Work out the finished part from the listing and answer in its coordinate system (mm). A direction names the side the tool comes from. Coordinates: 2 decimals unless noted, no trailing zeros. Order: outer loops, then holes, each group sorted by start corner. A loop starts at its lowest first (then second) coordinate and runs counter-clockwise, first axis right, second up. Notation, with made-up numbers: (42, -38.75) -> (58, -38.75) arc R21 cw to (58, -1.75) -> close; hole circle Ø3 at (67.25, -13). An arc over 180 degrees is marked (long way). Answer as CSV lines item,"result". Start each with the question number.
Item 1: Which of the six approach directions +Z, -Z, +X, -X, +Y, -Y give full straight-line access (tool end or side, diameter ignored) to faces 1 (the face through (-89.88, 10.61, 38.24)), 2 (the face through (-54, 3, 67.16)), 3 (the face through (-92.257, 5, 49))?
Item 2: For a pull along X with two mould halves and no side action, classify faces 4 (the face through (-93, 1.896, 60)), 5 (the face through (-55.257, 3, 62)), 6 (the face through (-92.257, 4, 60)) as pulls with the +X half, pulls with the -X half, needs draft (parallel to the pull), parting line crosses it, or undercut.
Item 3: Straight lines are drawn through the part: L1, parallel to Z at x = -71.5, y = 8; L2, parallel to X at y = 1.25, z = 71.5; L3, parallel to Z at x = -89, y = 6.25. For each, find the intervals that lie inside material, in ascending order.
Item 4: Section A-A (y = 15) is taken. Write down the section's boundary in (x, z).
Item 5: Section C-C (x = -68) is taken. Write down the section's boundary in (y, z).
Item 6: Each of these flat-tipped pins is pushed along its axis until it touches: pin 1 Ø2 at (y, z) = (11.5, 49) entering from -X; pin 2 Ø6 at (x, y) = (-65.5, 11.5) entering from +Z; pin 3 Ø4 at (x, z) = (-88, 46) entering from +Y. Where does it stop, or does it pass through?
Item 7: Section B-B (y = 11) is taken. Count the separate pieces of the cut face and the enclosed holes in it, then the cut area to 3 significant figures.
Autodesk Inventor part; units mm, degrees
ref_plane "YZ Plane" through (0, 0, 0) normal (1, 0, 0) x (0, 1, 0)
ref_plane "XZ Plane" through (0, 0, 0) normal (0, 1, 0) x (-1, 0, 0)
ref_plane "XY Plane" through (0, 0, 0) normal (0, 0, 1) x (1, 0, 0)
sketch "Sketch1" plane through (0, 0, 0) normal (0, 1, 0) x (-1, 0, 0)
  line L0 (94.2568, 73.4599) -> (94.2568, 30.8599)
  line L1 (94.2568, 30.8599) -> (50.7568, 30.8599)
  line L2 (50.7568, 30.8599) -> (50.7568, 73.4599)
  line L3 (50.7568, 73.4599) -> (94.2568, 73.4599)
  point P0 (0, 0)
  dimension "d0" = 42.6
  dimension "d1" = 43.5
extrude "Extrusion1" add sketch "Sketch1" along normal blind 1.6
sketch "Sketch2" plane through (0, 1.6, 0) normal (0, 1, 0) x (1, 0, 0)
  circle A0 centre (-53.6568, -70.5599) radius 1.5
  circle A1 centre (-53.6568, -33.9599) radius 1.5
  line L0 (-94.2568, -73.4599) -> (-50.7568, -73.4599)
  line L1 (-50.7568, -73.4599) -> (-50.7568, -30.8599)
  circle A2 centre (-91.6568, -33.9599) radius 1.5
  circle A3 centre (-91.6568, -70.5599) radius 1.5
  line L2 (-94.2568, -30.8599) -> (-94.2568, -73.4599)
  point P0 (0, 0)
  dimension "d4" = 3
  dimension "d5" = 3
  dimension "d6" = 36.6
  dimension "d7" = 2.9
  dimension "d8" = 2.9
  dimension "d9" = 2.9
  dimension "d10" = 3
  dimension "d11" = 38
  dimension "d12" = 3
  dimension "d13" = 38
  dimension "d14" = 2.6
extrude "Extrusion2" cut sketch "Sketch2" against normal blind 1.6
sketch "Sketch3" plane through (0, 1.6, 0) normal (0, 1, 0) x (1, 0, 0)
  line L0 (-65.7568, -67.8599) -> (-65.7568, -52.8599)
  line L1 (-65.7568, -51.8599) -> (-65.7568, -36.8599)
  line L2 (-50.7568, -73.4599) -> (-50.7568, -30.8599)
  line L3 (-65.7568, -67.8599) -> (-84.5568, -67.8599)
  line L4 (-84.5568, -67.8599) -> (-84.5568, -52.8599)
  line L5 (-84.5568, -52.8599) -> (-65.7568, -52.8599)
  line L6 (-65.7568, -51.8599) -> (-84.5568, -51.8599)
  line L7 (-84.5568, -51.8599) -> (-84.5568, -36.8599)
  line L8 (-84.5568, -36.8599) -> (-65.7568, -36.8599)
  line L9 (-94.2568, -73.4599) -> (-50.7568, -73.4599)
  point P0 (0, 0)
  dimension "d17" = 15
  dimension "d18" = 15
  dimension "d19" = 15
  dimension "d20" = 15
  dimension "d21" = 18.8
  dimension "d22" = 5.6
  dimension "d23" = 1
sketch "Sketch4" plane through (0, 1.6, 0) normal (0, 1, 0) x (1, 0, 0)
  line L0 (-55.2568, -67.1599) -> (-55.2568, -57.1599)
  line L1 (-55.2568, -57.1599) -> (-52.7568, -57.1599)
  line L2 (-52.7568, -57.1599) -> (-52.7568, -67.1599)
  line L3 (-52.7568, -67.1599) -> (-55.2568, -67.1599)
  line L4 (-50.7568, -73.4599) -> (-50.7568, -30.8599)
  line L5 (-94.2568, -73.4599) -> (-50.7568, -73.4599)
  point P0 (0, 0)
  dimension "d26" = 10
  dimension "d27" = 2
  dimension "d28" = 2.5
  dimension "d29" = 6.3
extrude "Extrusion4" add sketch "Sketch4" along normal blind 3
sketch "Sketch5" plane through (0, 4.6, 0) normal (0, 1, 0) x (1, 0, 0)
  circle A0 centre (-54.0568, -65.3099) radius 0.3
  circle A1 centre (-54.0568, -63.2099) radius 0.3
  circle A2 centre (-54.0568, -61.1099) radius 0.3
  circle A3 centre (-54.0568, -59.0099) radius 0.3
  line L0 (-55.2568, -67.1599) -> (-52.7568, -67.1599)
  line L1 (-52.7568, -67.1599) -> (-52.7568, -57.1599)
  point P0 (0, 0)
  dimension "d32" = 0.6
  dimension "d33" = 0.6
  dimension "d34" = 0.6
  dimension "d35" = 0.6
  dimension "d36" = 1.85
  dimension "d37" = 1.3
  dimension "d38" = 2.1
  dimension "d39" = 2.1
  dimension "d40" = 2.1
  dimension "d41" = 1.3
extrude "Extrusion5" add sketch "Sketch5" along normal blind 5.8
sketch "Sketch6" plane through (0, 1.6, 0) normal (0, 1, 0) x (1, 0, 0)
  circle A0 centre (-54.0568, -38.8599) radius 2
  circle A1 centre (-54.0568, -47.2599) radius 2
  circle A2 centre (-54.0568, -52.7599) radius 2
  circle A3 centre (-53.6568, -33.9599) radius 1.5
  line L0 (-50.7568, -30.8599) -> (-94.2568, -30.8599)
  line L1 (-50.7568, -30.8599) -> (-50.7568, -73.4599)
  point P0 (0, 0)
  dimension "d44" = 4
  dimension "d45" = 4
  dimension "d46" = 4
  dimension "d48" = 8
  dimension "d49" = 8.4
  dimension "d50" = 5.5
  dimension "d51" = 3.3
extrude "Extrusion6" add sketch "Sketch6" along normal blind 1.2 contours A0 | A1 | A2
sketch "Sketch7" plane through (-54.0568, 2.8, 52.7599) normal (0, 1, 0) x (1, 0, 0)
  circle A0 centre (0, 0) radius 2
  circle A1 centre (0, 0) radius 1.5
  point P0 (54.0568, 52.7599)
  dimension "d54" = 3
sketch "Sketch8" plane through (-54.0568, 2.8, 47.2599) normal (0, 1, 0) x (1, 0, 0)
  circle A0 centre (0, 0) radius 2
  circle A1 centre (0, 0) radius 1.5
  point P0 (54.0568, 47.2599)
  dimension "d55" = 3
sketch "Sketch9" plane through (-54.0568, 2.8, 38.8599) normal (0, 1, 0) x (1, 0, 0)
  circle A0 centre (0, 0) radius 2
  circle A1 centre (0, 0) radius 1.5
  point P0 (54.0568, 38.8599)
  dimension "d56" = 3
extrude "Extrusion7" add sketch "Sketch7" along normal blind 4.3 contours A1
extrude "Extrusion8" add sketch "Sketch8" along normal blind 4.3 contours A1
extrude "Extrusion9" add sketch "Sketch9" along normal blind 4.3 contours A1
fillet "Fillet1" radius 1.5 3 edges at (-55.5568, 7.1, 52.7599) (-55.5568, 7.1, 47.2599) (-55.5568, 7.1, 38.8599)
sketch "Sketch10" plane through (0, 1.6, 0) normal (0, 1, 0) x (1, 0, 0)
  line L0 (-85.2568, -36.9599) -> (-85.2568, -51.9599)
  line L1 (-85.2568, -51.9599) -> (-93.2568, -51.9599)
  line L2 (-93.2568, -51.9599) -> (-93.2568, -36.9599)
  line L3 (-93.2568, -36.9599) -> (-85.2568, -36.9599)
  line L4 (-93.2568, -52.9599) -> (-85.2568, -52.9599)
  line L5 (-85.2568, -52.9599) -> (-85.2568, -67.9599)
  line L6 (-85.2568, -67.9599) -> (-93.2568, -67.9599)
  line L7 (-93.2568, -67.9599) -> (-93.2568, -52.9599)
  line L8 (-84.5568, -36.8599) -> (-84.5568, -51.8599)
  line L9 (-50.7568, -30.8599) -> (-94.2568, -30.8599)
  point P0 (0, 0)
  dimension "d64" = 8
  dimension "d65" = 0.7
  dimension "d66" = 6.1
  dimension "d67" = 15
  dimension "d68" = 15
  dimension "d69" = 1
extrude "Extrusion10" add sketch "Sketch10" along normal blind 6
sketch "Sketch11" plane through (-93.2568, 1.6, 36.9599) normal (-1, 0, 0) x (0, 0, 1)
  line L0 (0.4, 0.8) -> (0.4, 5.8)
  line L1 (0.4, 5.8) -> (4.7, 5.8)
  line L2 (4.7, 5.8) -> (4.7, 0.8)
  line L3 (4.7, 0.8) -> (0.4, 0.8)
  line L4 (15, 0) -> (0, 0)
  line L5 (5.3, 5.8) -> (9.6, 5.8)
  line L6 (9.6, 5.8) -> (9.6, 0.8)
  line L7 (9.6, 0.8) -> (5.3, 0.8)
  line L8 (5.3, 0.8) -> (5.3, 5.8)
  line L9 (10.2, 5.8) -> (14.5, 5.8)
  line L10 (14.5, 5.8) -> (14.5, 0.8)
  line L11 (14.5, 0.8) -> (10.2, 0.8)
  line L12 (10.2, 0.8) -> (10.2, 5.8)
  line L13 (0, 0) -> (0, 6)
  point P0 (-36.9599, -1.6)
  dimension "d72" = 4.3
  dimension "d73" = 5
  dimension "d74" = 0.8
  dimension "d75" = 4.3
  dimension "d76" = 4.3
  dimension "d77" = 5
  dimension "d78" = 0.6
  dimension "d79" = 0.6
  dimension "d80" = 0.4
extrude "Extrusion11" cut sketch "Sketch11" against normal blind 1
sketch "Sketch12" plane through (0, 7.6, 0) normal (0, 1, 0) x (1, 0, 0)
  line L0 (-86.0568, -36.9599) -> (-91.0568, -36.9599)
  line L1 (-92.2568, -47.1599) -> (-92.2568, -51.4599)
  line L2 (-92.2568, -51.9599) -> (-86.0568, -51.9599)
  line L3 (-86.0568, -51.9599) -> (-86.0568, -36.9599)
  line L4 (-85.2568, -36.9599) -> (-93.2568, -36.9599)
  line L5 (-93.2568, -51.9599) -> (-85.2568, -51.9599)
  line L6 (-84.5568, -36.8599) -> (-84.5568, -51.8599)
  line L7 (-91.0568, -36.9599) -> (-91.0568, -51.9599)
  line L8 (-86.0568, -36.9599) -> (-91.0568, -36.9599)
  line L9 (-86.0568, -51.9599) -> (-91.0568, -51.9599)
  point P0 (0, 0)
  dimension "d83" = 0
  dimension "d84" = 0
  dimension "d85" = 1.5
  dimension "d86" = 5
extrude "Extrusion12" add sketch "Sketch12" along normal blind 4
ref_plane "Work Plane2" through (-91.0568, 11.6, 36.9599) normal (0.8762, -0.4819, 0) x (0, 0, 1)
sketch "Sketch13" plane through (-91.0568, 11.6, 36.9599) normal (0.8762, -0.4819, 0) x (0, 0, 1)
  line L0 (0, 0) -> (0, 4.5651)
  line L1 (0, 5.967) -> (0, 0.7097)
  line L2 (0, 4.5651) -> (15, 4.5651)
  line L3 (0, 4.5651) -> (15, 4.5651)
  line L4 (15, 4.5651) -> (15, 0)
  line L5 (15, 0) -> (0, 0)
  line L6 (0, 0) -> (15, 0)
  point P0 (-36.9599, -33.7179)
extrude "Extrusion13" add sketch "Sketch13" along normal blind 2
ref_plane "Work Plane3" through (-86.0568, 11.6, 51.9599) normal (-0.9806, -0.1961, 0) x (0, 0, -1)
sketch "Sketch14" plane through (-86.0568, 11.6, 51.9599) normal (-0.9806, -0.1961, 0) x (0, 0, -1)
  line L0 (15, 0) -> (15, 4.0792)
  line L1 (15, 4.0792) -> (0, 4.0792)
  line L2 (0, 4.0792) -> (0, 0)
  line L3 (0, 0) -> (15, 0)
  line L4 (0, 0) -> (15, 0)
  point P0 (51.9599, 28.2519)
extrude "Extrusion14" add sketch "Sketch14" along normal blind 2
sketch "Sketch15" plane through (0, 11.6, 0) normal (0, 1, 0) x (1, 0, 0)
  circle A0 centre (-88.5568, -39.4599) radius 1.8
  circle A1 centre (-88.5568, -44.4599) radius 1.8
  circle A2 centre (-88.5568, -49.4599) radius 1.8
  line L0 (-86.0568, -36.9599) -> (-91.0568, -36.9599)
  line L1 (-91.0568, -51.9599) -> (-86.0568, -51.9599)
  point P0 (0, 0)
  dimension "d93" = 3.6
  dimension "d94" = 3.6
  dimension "d95" = 3.6
  dimension "d96" = 2.5
  dimension "d97" = 5
  dimension "d98" = 5
extrude "Extrusion15" cut sketch "Sketch15" against normal blind 2
sketch "Sketch16" plane through (0, 7.6, 0) normal (0, 1, 0) x (1, 0, 0)
  line L0 (-85.2568, -52.9599) -> (-86.0568, -52.9599)
  line L1 (-85.2568, -52.9599) -> (-93.2568, -52.9599)
  line L2 (-86.0568, -51.9599) -> (-86.0568, -36.9599)
  line L3 (-86.0568, -52.9599) -> (-91.0568, -52.9599)
  line L4 (-91.0568, -52.9599) -> (-91.0568, -67.9599)
  line L5 (-93.2568, -67.9599) -> (-85.2568, -67.9599)
  line L6 (-86.0568, -52.9599) -> (-86.0568, -67.9599)
  line L7 (-91.0568, -67.9599) -> (-86.0568, -67.9599)
  point P0 (0, 0)
  dimension "d102" = 5
extrude "Extrusion16" add sketch "Sketch16" along normal blind 4
sketch "Sketch17" plane through (-91.0568, 11.6, 36.9599) normal (0.8762, -0.4819, 0) x (0, 0, 1)
  line L0 (16, 0) -> (16, 4.5662)
  line L1 (16, 4.5662) -> (31, 4.5662)
  line L2 (31, 5.967) -> (31, 0.7097)
  line L3 (31, 4.5662) -> (31, 0)
  line L4 (31, 1.0953) -> (31, -2.4096)
  line L5 (31, 0) -> (16, 0)
  line L6 (16, 0) -> (31, 0)
  point P0 (-36.9599, -33.7179)
extrude "Extrusion17" add sketch "Sketch17" along normal blind 4
sketch "Sketch18" plane through (-86.0568, 11.6, 51.9599) normal (-0.9806, -0.1961, 0) x (0, 0, -1)
  line L0 (-1, 4.0792) -> (-1, 0)
  line L1 (-1, 0) -> (-16, 0)
  line L2 (-16, 0) -> (-1, 0)
  line L3 (-16, 0) -> (-16, 4.0792)
  line L4 (-16, 3.9223) -> (-16, 0)
  line L5 (-16, 4.0792) -> (-1, 4.0792)
  line L6 (-16, 4.0792) -> (-1, 4.0792)
  point P0 (51.9599, 28.2519)
extrude "Extrusion18" add sketch "Sketch18" along normal blind 4
sketch "Sketch19" plane through (0, 11.6, 0) normal (0, 1, 0) x (1, 0, 0)
  circle A0 centre (-88.5568, -55.4599) radius 1.8
  circle A1 centre (-88.5568, -60.4599) radius 1.8
  circle A2 centre (-88.5568, -65.4599) radius 1.8
  line L0 (-86.0568, -52.9599) -> (-91.0568, -52.9599)
  line L1 (-91.0568, -67.9599) -> (-86.0568, -67.9599)
  line L2 (-91.0568, -52.9599) -> (-91.0568, -67.9599)
  point P0 (0, 0)
  dimension "d109" = 3.6
  dimension "d110" = 3.6
  dimension "d111" = 3.6
  dimension "d112" = 2.5
  dimension "d113" = 1.4
  dimension "d115" = 1.4
  dimension "d116" = 2.5
  dimension "d117" = 2.5
  dimension "d118" = 2.5
extrude "Extrusion19" cut sketch "Sketch19" against normal blind 2
sketch "Sketch20" plane through (-93.2568, 1.6, 52.9599) normal (-1, 0, 0) x (0, 0, 1)
  line L0 (0.4, 5.2955) -> (4.7, 5.2955)
  line L1 (4.7, 5.2955) -> (4.7, 0.2955)
  line L2 (4.7, 0.2955) -> (0.4, 0.2955)
  line L3 (0.4, 0.2955) -> (0.4, 5.2955)
  line L4 (5.3, 5.2955) -> (9.6, 5.2955)
  line L5 (9.6, 5.2955) -> (9.6, 0.2955)
  line L6 (9.6, 0.2955) -> (5.3, 0.2955)
  line L7 (5.3, 0.2955) -> (5.3, 5.2955)
  line L8 (10.2, 5.2955) -> (14.5, 5.2955)
  line L9 (14.5, 5.2955) -> (14.5, 0.2955)
  line L10 (14.5, 0.2955) -> (10.2, 0.2955)
  line L11 (10.2, 0.2955) -> (10.2, 5.2955)
  line L12 (0, 0) -> (0, 5.9988)
  point P0 (-52.9599, -1.6)
  dimension "d121" = 4.3
  dimension "d122" = 5
  dimension "d123" = 4.3
  dimension "d124" = 5
  dimension "d125" = 4.3
  dimension "d126" = 5
  dimension "d127" = 0.4
  dimension "d128" = 0.6
  dimension "d129" = 0.6
extrude "Extrusion20" cut sketch "Sketch20" against normal blind 1
extrude "Extrusion21" add sketch "Sketch3" along normal blind 15.7
chamfer "Chamfer1" distance 1 angle 45 4 edges at (-94.2568, 0.8, 30.8599) (-50.7568, 0.8, 30.8599) (-94.2568, 0.8, 73.4599) (-50.7568, 0.8, 73.4599)
fillet "Fillet2" radius 0.2 3 edges at (-56.0568, 2.8, 52.7599) (-56.0568, 2.8, 47.2599) (-56.0568, 2.8, 38.8599)
sketch "Sketch21" plane through (0, 1.6, 0) normal (0, 1, 0) x (1, 0, 0)
  circle A0 centre (-53.6568, -70.5599) radius 1.5
  circle A1 centre (-53.6568, -70.5599) radius 1.5
  circle A2 centre (-91.6568, -70.5599) radius 1.5
  circle A3 centre (-91.6568, -70.5599) radius 1.5
  circle A4 centre (-53.6568, -33.9599) radius 1.5
  circle A5 centre (-53.6568, -33.9599) radius 1.5
  circle A6 centre (-91.6568, -33.9599) radius 1.5
  circle A7 centre (-91.6568, -33.9599) radius 1.5
  point P0 (0, 0)
equation "\"d41\" = d37"
equation "\"d117\" = d116"
equation "\"d118\" = d116"
properties part number "relay_module"
Checked values:
1,face 1,"+Y"
1,face 2,"+Z, +X, +Y"
1,face 3,"-X"
2,face 4,"needs draft"
2,face 5,"undercut"
2,face 6,"pulls with the -X half"
3,L1,"z = 36.86 to 51.86, 52.86 to 67.86"
3,L2,"x = -94.26 to -92.83, -90.49 to -54.83, -52.49 to -50.76"
3,L3,"z = 36.96 to 51.96, 52.96 to 67.96"
4,outline,"(-84.56, 36.86) -> (-65.76, 36.86) -> (-65.76, 51.86) -> (-84.56, 51.86) -> close; (-84.56, 52.86) -> (-65.76, 52.86) -> (-65.76, 67.86) -> (-84.56, 67.86) -> close"
5,outline,"(0, 30.86) -> (1.6, 30.86) -> (1.6, 36.86) -> (17.3, 36.86) -> (17.3, 51.86) -> (1.6, 51.86) -> (1.6, 52.86) -> (17.3, 52.86) -> (17.3, 67.86) -> (1.6, 67.86) -> (1.6, 73.46) -> (0, 73.46) -> close"
6,pin 1,"stops at x = -91.66"
6,pin 2,"stops at z = 67.86"
6,pin 3,"stops at y = 11.6"
7,separate pieces,"4"
7,enclosed holes,"6"
7,area,"666 mm^2"
